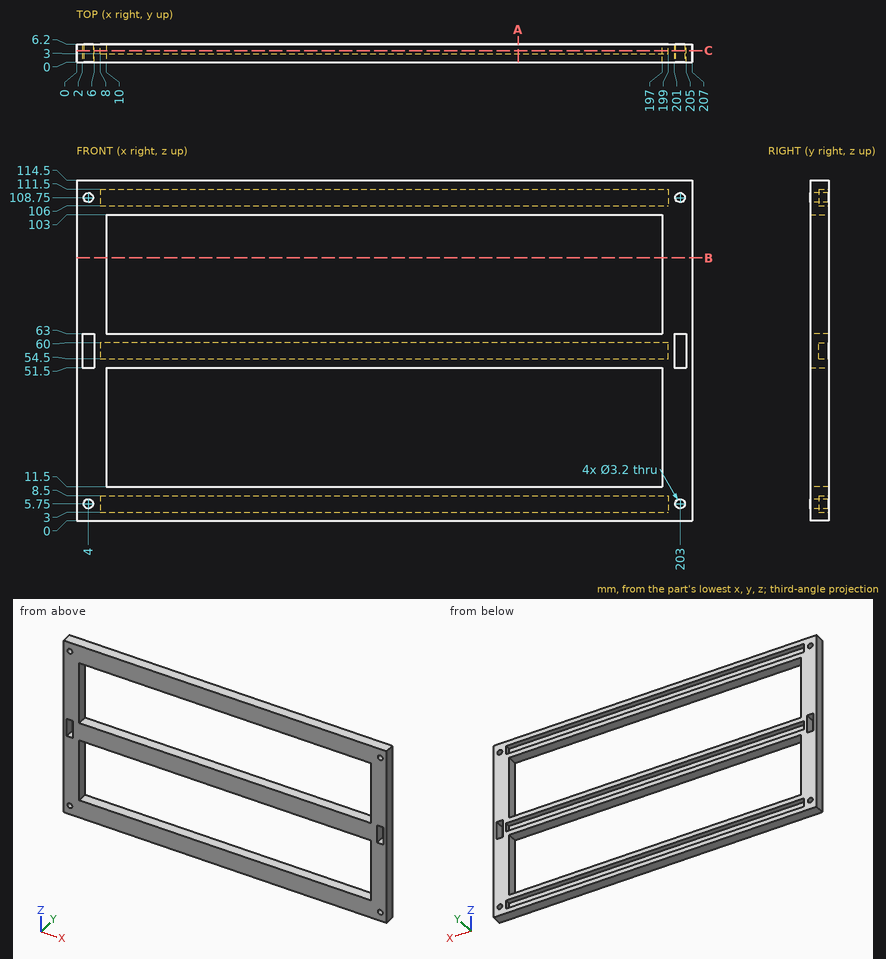
Design review of the part shown in the three views and the two pictorial views. Dimensions are in mm from the part's minimum x, y and z. Give positions to 0.01 mm unless a question says otherwise; leave off trailing zeros. Order: outer loops, then holes, each group sorted by start corner. A loop starts at its lowest first (then second) coordinate and runs counter-clockwise, first axis right, second up. Notation, with made-up numbers: M 81,4 L 110,4 A20 cw 110,12 Z; hole C 78,30.25 d8. An arc over 180 degrees is marked long. Answer in a Markdown table with one row per item. Add a question column.
(1) Wall thickness on probe 1 along X at (y, z) = (2.75, 108.75); probe 2 along Z at (x, y) = (4, 3.75); probe 3 along Z at (x, y) = (87, 4.75): over which ranges is each line inside the solid? List them lowest first. Write a range as [from, to].
(2) Consider section C-C on y = 4. Give the number of separate pieces and of enclosed holes in the cut face, and give its area (3 significant figures).
(3) Consider section B-B on z = 88.5. State the section outline as (x, y) points.
(4) For pin 1 (1.6 mm diameter, centred on x = 89, z = 5, fed in from +Y), flat-tipped, find the tip position at first contact; note if it passes through.
(5) Consider section A-A on x = 148.5. State the section outline as (y, z) points.
Evaluation:
| question | item | result |
|---|---|---|
| 1 | probe 1 | x = [0, 2.4], [5.6, 201.4], [204.6, 207] |
| 1 | probe 2 | z = [0, 4.15], [7.35, 51.5], [63, 107.15], [110.35, 114.5] |
| 1 | probe 3 | z = [0, 3], [8.5, 11.5], [51.5, 54.5], [60, 63], [103, 106], [111.5, 114.5] |
| 2 | separate pieces | 1 |
| 2 | enclosed holes | 11 |
| 2 | area | 5,470 mm^2 |
| 3 | outline | M 0,0 L 10,0 L 10,6.2 L 0,6.2 Z; M 197,0 L 207,0 L 207,6.2 L 197,6.2 Z |
| 4 | pin 1 | stops at y = 3 |
| 5 | outline | M 0,0 L 6.2,0 L 6.2,3 L 3,3 L 3,8.5 L 6.2,8.5 L 6.2,11.5 L 0,11.5 Z; M 0,51.5 L 6.2,51.5 L 6.2,54.5 L 3,54.5 L 3,60 L 6.2,60 L 6.2,63 L 0,63 Z; M 0,103 L 6.2,103 L 6.2,106 L 3,106 L 3,111.5 L 6.2,111.5 L 6.2,114.5 L 0,114.5 Z |
